```python
from build123d import *

# Parameters (mm, degrees)
F0_W     = 81
F0_H     = 36
F1_DEPTH = 35
F2_W     = 71
F2_H     = 26
F3_DEPTH = 35.001
F4_R     = 1.65
F5_DEPTH = 35.001


with BuildPart() as f1:
    # F0 (on Front) → F1 (new body)
    with BuildSketch(Plane.XZ):
        Rectangle(F0_W, F0_H)
    extrude(amount=F1_DEPTH)

    # F2 (on face) → F3 (cut, through all)
    with BuildSketch(Plane.XZ.offset(35)):
        Rectangle(F2_W, F2_H)
    extrude(amount=-F3_DEPTH, mode=Mode.SUBTRACT)

    # F4 (on face) → F5 (cut, through all)
    with BuildSketch(Plane.XZ.offset(35)):
        with Locations((0, 15.5)):
            Circle(F4_R)
        with Locations((38, 15.5)):
            Circle(F4_R)
        with Locations((38, 0)):
            Circle(F4_R)
        with Locations((38, -15.5)):
            Circle(F4_R)
        with Locations((0, -15.5)):
            Circle(F4_R)
        with Locations((-38, -15.5)):
            Circle(F4_R)
        with Locations((-38, 0)):
            Circle(F4_R)
        with Locations((-38, 15.5)):
            Circle(F4_R)
    extrude(amount=-F5_DEPTH, mode=Mode.SUBTRACT)


solid = f1.part
```
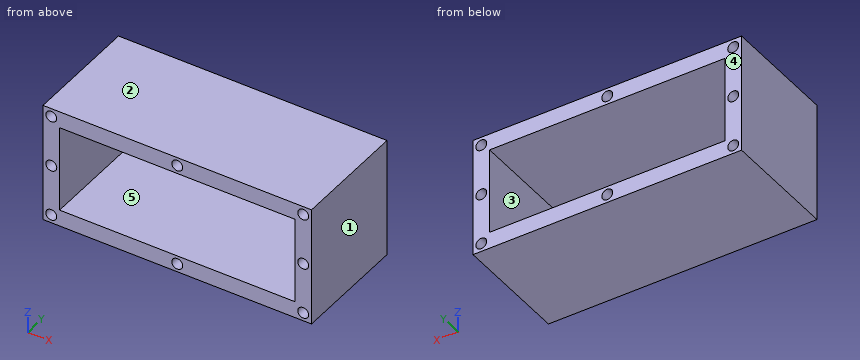
Geometry: final body of the model. Coordinates: model frame, mm. Face numbers are marked on the shaded views. A direction names the side the tool comes from. Round coordinates to 2 decimals unless told otherwise and drop trailing zeros. Write each loop counter-clockwise with the first axis right and the second up, starting at its lowest first coordinate (ties: lowest second). Pieces come first, ordered by that corner, then holes.
Item 1: Section query B-B (z = -15.5). Return loops of the section in (x, y), plus the area to 3 significant figures.
Item 2: Section query D-D (z = -10.5). Return loops of the section in (x, y), plus the area to 3 significant figures.
Item 3: Mould query, pull axis X, two halves, no side actions, for the marked faces 1, 2 and 3. Classes: +X half, -X half, draft (parallel to the pull), parting line (faces both ways), or undercut.
Item 4: Section query C-C (y = -28.5). Give the number of separate pieces and of enclosed holes in the cut face, plus the area to 3 significant figures.
Item 5: Section query A-A (x = 0). Return loops of the section in (y, z), plus the area to 3 significant figures.
Item 6: Material intervals for L1, parallel to Z at x = -38, y = -19; L2, parallel to Z at x = 10, y = -13; L3, parallel to Z at x = 0, y = -17, sorted ascending.
Item 7: Pin query (flat end, axial travel): P1, Ø5.5, axis at x = 38, z = 15.5, coming from the +Y side; P2, Ø3, axis at x = 0, z = 15.5, coming from the +Y side. Return the tip coordinate at first contact, or that it passes through.
Item 8: Set-up query: the marked faces 4 and 5. Return all of +Z, -Z, +X, -X, +Y, -Y with unobstructed straight access to the full face (end or side cutting, diameter ignored); none if empty.
Completed:
1. outline: (-40.5, -35) - (-39.65, -35) - (-39.65, 0) - (-40.5, 0) - close; (-36.35, -35) - (-1.65, -35) - (-1.65, 0) - (-36.35, 0) - close; (1.65, -35) - (36.35, -35) - (36.35, 0) - (1.65, 0) - close; (39.65, -35) - (40.5, -35) - (40.5, 0) - (39.65, 0) - close
1. area: 2,490 mm2
2. outline: (-40.5, -35) - (-35.5, -35) - (-35.5, 0) - (-40.5, 0) - close; (35.5, -35) - (40.5, -35) - (40.5, 0) - (35.5, 0) - close
2. area: 350 mm2
3. face 1: +X half
3. face 2: draft
3. face 3: undercut
4. separate pieces: 1
4. enclosed holes: 9
4. area: 1,000 mm2
5. outline: (-35, -18) - (0, -18) - (0, -17.15) - (-35, -17.15) - close; (-35, -13.85) - (0, -13.85) - (0, -13) - (-35, -13) - close; (-35, 13) - (0, 13) - (0, 13.85) - (-35, 13.85) - close; (-35, 17.15) - (0, 17.15) - (0, 18) - (-35, 18) - close
5. area: 119 mm2
6. L1: z = -18 to -17.15, -13.85 to -1.65, 1.65 to 13.85, 17.15 to 18
6. L2: z = -18 to -13, 13 to 18
6. L3: z = -18 to -17.15, -13.85 to -13, 13 to 13.85, 17.15 to 18
7. P1: stops at y = 0
7. P2: passes through
8. face 4: +Z, -Z, +X, -X, +Y
8. face 5: +Y, -Y
